Source: CAD feature listing. Evaluate the final solid. Frame: model axes, mm. Round coordinates to 2 decimals unless told otherwise and drop trailing zeros. Order: outer loops, then holes, each group sorted by start corner. A loop starts at its lowest first (then second) coordinate and runs counter-clockwise, first axis right, second up. Notation, with made-up numbers: (18, 19.25) -> (73, 19.25) arc R36 ccw to (73, 58.25) -> close; hole circle Ø4 at (56, -13.5). An arc over 180 degrees is marked (long way). Write item = value, one per line. Start each with the question number.
(1) Cut plane A-A on x = -7. Return the cut outline in (y, z).
(2) Ray query, line 1 (Y direction, x = -15.5, z = 2.4); line 2 (X direction, y = -139.5, z = 3.9). Return the intervals inside material, ascending.
(3) Contact query for flat-ended pins moving along their axis: pin 1 Ø1.2 at (y, z) = (-288.5, 2) entering from +X; pin 2 Ø2 at (x, z) = (338.5, 1.5) entering from +Y; pin 3 Ø1.2 at (y, z) = (289, 1) entering from +X. Output: stop coordinate, or through.
from build123d import *

# Parameters (mm, degrees)
SKETCH1_W           = 70
SKETCH1_H           = 4
SKETCH1_W_2         = 4
SKETCH1_H_2         = 70
BOSS_EXTRUDE1_DEPTH = 4.3


with BuildPart() as part:
    # Sketch1 → Boss-Extrude1 (new body)
    with BuildSketch(Plane.XY):
        with BuildLine():
            Line((-325, -300), (325, -300))
            ThreePointArc((325, -300), (342.67766953, -292.67766953), (350, -275))
            Line((350, -275), (350, 275))
            ThreePointArc((350, 275), (342.67766953, 292.67766953), (325, 300))
            Line((325, 300), (-325, 300))
            ThreePointArc((-325, 300), (-342.67766953, 292.67766953), (-350, 275))
            Line((-350, 275), (-350, -275))
            ThreePointArc((-350, -275), (-342.67766953, -292.67766953), (-325, -300))
        make_face()
        with Locations((-240, -288)):
            Rectangle(SKETCH1_W, SKETCH1_H, mode=Mode.SUBTRACT)
        with Locations((338, -111.6666)):
            Rectangle(SKETCH1_W_2, SKETCH1_H_2, mode=Mode.SUBTRACT)
        with Locations((338, 111.6667)):
            Rectangle(SKETCH1_W_2, SKETCH1_H_2, mode=Mode.SUBTRACT)
        with Locations((0, -288)):
            Rectangle(SKETCH1_W, SKETCH1_H, mode=Mode.SUBTRACT)
        with Locations((240, -288)):
            Rectangle(SKETCH1_W, SKETCH1_H, mode=Mode.SUBTRACT)
        with Locations((-338, 111.6667)):
            Rectangle(SKETCH1_W_2, SKETCH1_H_2, mode=Mode.SUBTRACT)
        with Locations((-338, -111.6666)):
            Rectangle(SKETCH1_W_2, SKETCH1_H_2, mode=Mode.SUBTRACT)
        with Locations((120, 111.6667)):
            Rectangle(SKETCH1_W_2, SKETCH1_H_2, mode=Mode.SUBTRACT)
        with Locations((-120, -111.6667)):
            Rectangle(SKETCH1_W_2, SKETCH1_H_2, mode=Mode.SUBTRACT)
        with Locations((0, 111.6667)):
            Rectangle(SKETCH1_W, SKETCH1_H, mode=Mode.SUBTRACT)
        with Locations((-240, 111.6667)):
            Rectangle(SKETCH1_W, SKETCH1_H, mode=Mode.SUBTRACT)
        with Locations((240, 111.6667)):
            Rectangle(SKETCH1_W, SKETCH1_H, mode=Mode.SUBTRACT)
        with Locations((-240, -111.6667)):
            Rectangle(SKETCH1_W, SKETCH1_H, mode=Mode.SUBTRACT)
        with Locations((0, -111.6667)):
            Rectangle(SKETCH1_W, SKETCH1_H, mode=Mode.SUBTRACT)
        with Locations((240, -111.6667)):
            Rectangle(SKETCH1_W, SKETCH1_H, mode=Mode.SUBTRACT)
        with Locations((-240, 288)):
            Rectangle(SKETCH1_W, SKETCH1_H, mode=Mode.SUBTRACT)
        with Locations((0, 288)):
            Rectangle(SKETCH1_W, SKETCH1_H, mode=Mode.SUBTRACT)
        with Locations((240, 288)):
            Rectangle(SKETCH1_W, SKETCH1_H, mode=Mode.SUBTRACT)
    extrude(amount=BOSS_EXTRUDE1_DEPTH)


solid = part.part
Evaluation:
q1.outline = (-300, 0) -> (-290, 0) -> (-290, 4.3) -> (-300, 4.3) -> close; (-286, 0) -> (-113.67, 0) -> (-113.67, 4.3) -> (-286, 4.3) -> close; (-109.67, 0) -> (109.67, 0) -> (109.67, 4.3) -> (-109.67, 4.3) -> close; (113.67, 0) -> (286, 0) -> (286, 4.3) -> (113.67, 4.3) -> close; (290, 0) -> (300, 0) -> (300, 4.3) -> (290, 4.3) -> close
q2.line_1 = -300 to -290, -286 to -113.67, -109.67 to 109.67, 113.67 to 286, 290 to 300
q2.line_2 = -350 to -340, -336 to -122, -118 to 336, 340 to 350
q3.pin_1 = 346.41
q3.pin_2 = 296.65
q3.pin_3 = 346.11
